```python
from build123d import *

# Parameters (mm, degrees)
EXTRUDE_1_DEPTH      = 4.7
EXTRUDE_1_DEPTH_BACK = 4.7
SKETCH_1_W           = 25.3
SKETCH_1_H           = 39.12
SKETCH_2_W           = 9
SKETCH_2_H           = 7.4
CUT_EXTRUDE_2_DEPTH  = 10
SKETCH_3_W           = 9
SKETCH_3_H           = 7.4
EXTRUDE_4_DEPTH      = 0.1
SKETCH_4_R           = 0.65
SKETCH_4_R_2         = 0.4
EXTRUDE_3_DEPTH      = 4.2


with BuildPart() as part:
    # Sketch 1 → Extrude 1 (new, two sides: drawn at the far end of the back side and taken through both)
    with BuildSketch(Plane(origin=(0, 0, 0), x_dir=(1, 0, 0), z_dir=(0, 1, 0)).offset(-EXTRUDE_1_DEPTH_BACK)):
        Rectangle(SKETCH_1_W, SKETCH_1_H)
    extrude(amount=EXTRUDE_1_DEPTH + EXTRUDE_1_DEPTH_BACK)

    # Sketch 2 → Cut-Extrude 2 (cut)
    with BuildSketch(Plane.XY.offset(19.56)):
        with Locations((-6.95, 0)):
            Rectangle(SKETCH_2_W, SKETCH_2_H)
    extrude(amount=-CUT_EXTRUDE_2_DEPTH, mode=Mode.SUBTRACT)

    # Sketch 3 → Extrude 4 (add)
    with BuildSketch(Plane.XY.offset(19.56)):
        with Locations((6.95, 0)):
            Rectangle(SKETCH_3_W, SKETCH_3_H)
    extrude(amount=EXTRUDE_4_DEPTH)

    # Sketch 4 → Extrude 3 (add)
    with BuildSketch(Plane.XZ.offset(4.7)):
        with Locations(Location((-10.16, 3.36, 0), (0, 0, 90))):
            Circle(SKETCH_4_R)
        with Locations(Location((10.16, 3.36, 0), (0, 0, 90))):
            Circle(SKETCH_4_R)
        with Locations(Location((-10.16, -16.64, 0), (0, 0, 90))):
            Circle(SKETCH_4_R_2)
        with Locations(Location((-7.62, -16.64, 0), (0, 0, 90))):
            Circle(SKETCH_4_R_2)
        with Locations(Location((-5.08, -16.64, 0), (0, 0, 90))):
            Circle(SKETCH_4_R_2)
        with Locations(Location((-2.54, -16.64, 0), (0, 0, 90))):
            Circle(SKETCH_4_R_2)
        with Locations(Location((0, -16.64, 0), (0, 0, 90))):
            Circle(SKETCH_4_R_2)
        with Locations(Location((2.54, -16.64, 0), (0, 0, 90))):
            Circle(SKETCH_4_R_2)
        with Locations(Location((5.08, -16.64, 0), (0, 0, 90))):
            Circle(SKETCH_4_R_2)
        with Locations(Location((7.62, -16.64, 0), (0, 0, 90))):
            Circle(SKETCH_4_R_2)
        with Locations(Location((10.16, -16.64, 0), (0, 0, 90))):
            Circle(SKETCH_4_R_2)
    extrude(amount=EXTRUDE_3_DEPTH)


solid = part.part
```
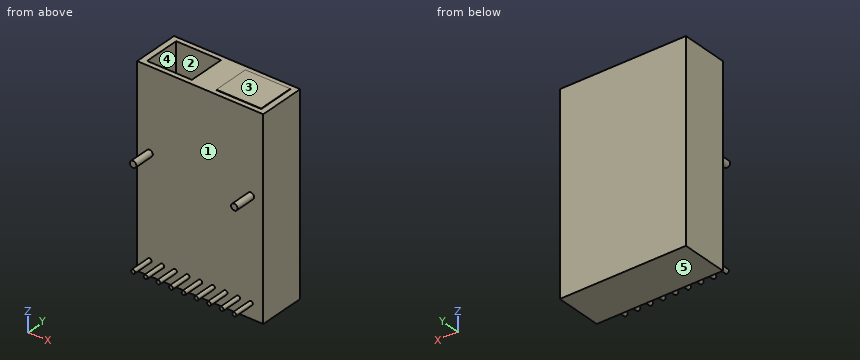
Source: CAD feature listing. Evaluate the final solid. Frame: model axes, mm. Face numbers are marked on the shaded views. A direction names the side the tool comes from. Coordinates: 2 decimals unless noted, no trailing zeros. Order: outer loops, then holes, each group sorted by start corner. A loop starts at its lowest first (then second) coordinate and runs counter-clockwise, first axis right, second up. Notation, with made-up numbers: (49, -14.75) - (87, -14.75) arc R23 cw to (87, 15.25) - close; hole circle Ø11 at (15.25, 26.25). An arc over 180 degrees is marked (long way). One line per item, written item: value.
1) Contact query for flat-ended pins moving along their axis: pin 1 (6 mm diameter, centred on x = 9.5, y = -7, fed in from +Z); pin 2 (5 mm diameter, centred on x = 2, y = -5.5, fed in from -Z); pin 3 (4 mm diameter, centred on x = 6.5, z = 9, fed in from -Y). Output: stop coordinate, or through.
Computed values:
pin 1: stops at z = 19.56
pin 2: stops at z = -19.56
pin 3: stops at y = -4.7
2) Cut plane D-D on y = 1.75. Output: boundary loops of the cut face in (x, z), plus the area to 3 significant figures.
Computed values:
outline: (-12.65, -19.56) - (12.65, -19.56) - (12.65, 19.56) - (11.45, 19.56) - (11.45, 19.66) - (2.45, 19.66) - (2.45, 19.56) - (-2.45, 19.56) - (-2.45, 9.56) - (-11.45, 9.56) - (-11.45, 19.56) - (-12.65, 19.56) - close
area: 901 mm^2
3) Ray query, line 1 (X direction, y = -3.25, z = 14); line 2 (Y direction, x = -3, z = 11); line 3 (Y direction, x = 7.5, z = -18). Return the intervals inside material, ascending. Write a range as [from, to].
Computed values:
line 1: x = [-12.65, -11.45], [-2.45, 12.65]
line 2: y = [-4.7, -3.7], [3.7, 4.7]
line 3: y = [-4.7, 4.7]
4) Cut plane B-B on z = 10. Output: boundary loops of the cut face in (x, y), plus the area to 3 significant figures.
Computed values:
outline: (-12.65, -4.7) - (12.65, -4.7) - (12.65, 4.7) - (-12.65, 4.7) - close; hole (-11.45, -3.7) - (-2.45, -3.7) - (-2.45, 3.7) - (-11.45, 3.7) - close
area: 171 mm^2
5) Cut plane C-C on x = 10.16. Output: boundary loops of the cut face in (y, z).
Computed values:
outline: (-8.9, -17.04) - (-4.7, -17.04) - (-4.7, -19.56) - (4.7, -19.56) - (4.7, 19.56) - (3.7, 19.56) - (3.7, 19.66) - (-3.7, 19.66) - (-3.7, 19.56) - (-4.7, 19.56) - (-4.7, 4.01) - (-8.9, 4.01) - (-8.9, 2.71) - (-4.7, 2.71) - (-4.7, -16.24) - (-8.9, -16.24) - close
6) Reachability of the marked faces 4 and 5 from +Z, -Z, +X, -X, +Y, -Y: full face, straight path, thin tool, end or side. Return the list, or none.
Computed values:
face 4: +Z
face 5: -Z, +X, -X, +Y, -Y
7) Cut plane A-A on y = -7.5. State how many separate pieces and enclosed holes the cut face has, plus the area to 3 significant figures.
Computed values:
separate pieces: 11
enclosed holes: 0
area: 7.18 mm^2
8) Mould query, pull axis Y, two halves, no side actions, for the marked faces 1, 2 and 3. Classes: released by +Y, released by -Y, zero draft, split by the parting line, or undercut.
Computed values:
face 1: released by -Y
face 2: undercut
face 3: zero draft
